Autodesk Inventor part; units mm, degrees
ref_plane "YZ Plane" through (0, 0, 0) normal (1, 0, 0) x (0, 1, 0)
ref_plane "XZ Plane" through (0, 0, 0) normal (0, 1, 0) x (-1, 0, 0)
ref_plane "XY Plane" through (0, 0, 0) normal (0, 0, 1) x (1, 0, 0)
sketch "Sketch1" plane through (0, 0, 0) normal (0, 0, 1) x (1, 0, 0)
  circle A0 centre (0, 0) radius 3.5
  line L0 (77.9423, 0) -> (38.9711, -67.5)
  line L1 (38.9711, -67.5) -> (-38.9711, -67.5)
  line L2 (-38.9711, -67.5) -> (-77.9423, 0)
  line L3 (-77.9423, 0) -> (-38.9711, 67.5)
  line L4 (-38.9711, 67.5) -> (38.9711, 67.5)
  line L5 (38.9711, 67.5) -> (77.9423, 0)
  circle A1 centre (22.5, 0) radius 2.25
  circle A2 centre (54, 0) radius 2
  circle A3 centre (15.9099, 15.9099) radius 2.25
  circle A4 centre (0, 22.5) radius 2.25
  circle A5 centre (-15.9099, 15.9099) radius 2.25
  circle A6 centre (-22.5, 0) radius 2.25
  circle A7 centre (-15.9099, -15.9099) radius 2.25
  circle A8 centre (0, -22.5) radius 2.25
  circle A9 centre (15.9099, -15.9099) radius 2.25
  circle A10 centre (46.7654, 27) radius 2
  circle A11 centre (27, 46.7654) radius 2
  circle A12 centre (0, 54) radius 2
  circle A13 centre (-27, 46.7654) radius 2
  circle A14 centre (-46.7654, 27) radius 2
  circle A15 centre (-54, 0) radius 2
  circle A16 centre (-46.7654, -27) radius 2
  circle A17 centre (-27, -46.7654) radius 2
  circle A18 centre (0, -54) radius 2
  circle A19 centre (27, -46.7654) radius 2
  circle A20 centre (46.7654, -27) radius 2
  dimension "d0" = 7
  dimension "d1" = 135
  dimension "d2" = 22.5
  dimension "d3" = 4.5
  dimension "d4" = 4
  dimension "d5" = 54
  dimension "d8" = 360
  dimension "d12" = 360
extrude "Extrusion1" add sketch "Sketch1" along normal blind 30
sketch "Sketch2" plane through (0, 0, 30) normal (0, 0, 1) x (1, 0, 0)
  circle A0 centre (0, 0) radius 3.5
  circle A1 centre (0, 0) radius 49
  dimension "d16" = 98
extrude "Extrusion2" cut sketch "Sketch2" against normal blind 15
sketch "Sketch3" plane through (0, 0, 15) normal (0, 0, 1) x (1, 0, 0)
  circle A0 centre (0, 0) radius 33
  dimension "d19" = 66
extrude "Extrusion3" cut sketch "Sketch3" against normal blind 3
sketch "Sketch4" plane through (0, 0, 12) normal (0, 0, 1) x (1, 0, 0)
  circle A0 centre (0, 0) radius 16.5
  circle A1 centre (0, 0) radius 3.5
  dimension "d22" = 33
extrude "Extrusion4" add sketch "Sketch4" along normal blind 33
sketch "Sketch5" plane through (0, 0, 45) normal (0, 0, 1) x (1, 0, 0)
  circle A0 centre (8, 0) radius 2.5
  circle A1 centre (2.4721, 7.6085) radius 2.5
  circle A2 centre (-6.4721, 4.7023) radius 2.5
  circle A3 centre (-6.4721, -4.7023) radius 2.5
  circle A4 centre (2.4721, -7.6085) radius 2.5
  point P0 (0, 0)
  dimension "d25" = 5
  dimension "d26" = 8
  dimension "d29" = 360
extrude "Extrusion5" cut sketch "Sketch5" against normal through all
sketch "Sketch6" plane through (0, 0, 0) normal (0, 0, -1) x (-1, 0, 0)
  circle A0 centre (0, 0) radius 17.5
  dimension "d33" = 35
extrude "Extrusion6" cut sketch "Sketch6" against normal blind 5
sketch "Sketch10" plane through (0, 0, 0) normal (0, 0, -1) x (-1, 0, 0)
  circle A0 centre (22.5, 0) radius 2.25
  circle A1 centre (0, 0) radius 3.5
  circle A2 centre (0, 0) radius 20.25
  circle A3 centre (0, 0) radius 24.75
  circle A4 centre (0, 0) radius 16
  circle A5 centre (0, 0) radius 29
  line L0 (29, 0) -> (16, 0)
  dimension "d38" = 13
extrude "Extrusion7" cut sketch "Sketch10" against normal blind 5 contours L0 A0 | A2 | A3 | A5 | A0 L0
sketch "Sketch11" plane through (0, 0, 12) normal (0, 0, 1) x (1, 0, 0)
  circle A0 centre (0, 0) radius 16.5
  circle A1 centre (15.9099, -15.9099) radius 2.25
  circle A2 centre (0, -22.5) radius 2.25
  circle A3 centre (-15.9099, -15.9099) radius 2.25
  circle A4 centre (-22.5, 0) radius 2.25
  circle A5 centre (-15.9099, 15.9099) radius 2.25
  circle A6 centre (0, 22.5) radius 2.25
  circle A7 centre (15.9099, 15.9099) radius 2.25
  circle A8 centre (22.5, 0) radius 2.25
  circle A9 centre (0, 0) radius 33
extrude "Extrusion8" add sketch "Sketch11" along normal up to surface (3 mm away) from surface at 0
sketch "Sketch12" plane through (0, 0, 30) normal (0, 0, 1) x (1, 0, 0)
  circle A0 centre (0, 0) radius 49
  circle A1 centre (46.7654, -27) radius 2
  circle A2 centre (27, -46.7654) radius 2
  circle A3 centre (0, -54) radius 2
  circle A4 centre (-27, -46.7654) radius 2
  circle A5 centre (-46.7654, -27) radius 2
  circle A6 centre (-54, 0) radius 2
  circle A7 centre (-46.7654, 27) radius 2
  circle A8 centre (-27, 46.7654) radius 2
  circle A9 centre (0, 54) radius 2
  circle A10 centre (27, 46.7654) radius 2
  circle A11 centre (46.7654, 27) radius 2
  circle A12 centre (54, 0) radius 2
  line L0 (38.9711, -67.5) -> (77.9423, 0)
  line L1 (77.9423, 0) -> (38.9711, 67.5)
  line L2 (38.9711, 67.5) -> (-38.9711, 67.5)
  line L3 (-38.9711, 67.5) -> (-77.9423, 0)
  line L4 (-77.9423, 0) -> (-38.9711, -67.5)
  line L5 (-38.9711, -67.5) -> (38.9711, -67.5)
extrude "Extrusion9" cut sketch "Sketch12" against normal blind 1
sketch "Sketch14" plane through (0, 0, 15) normal (0, 0, 1) x (1, 0, 0)
  circle A0 centre (0, 0) radius 3.5
  circle A1 centre (0, 0) radius 33
  circle A2 centre (15.9099, -15.9099) radius 2.25
  circle A3 centre (0, -22.5) radius 2.25
  circle A4 centre (-15.9099, -15.9099) radius 2.25
  circle A5 centre (-22.5, 0) radius 2.25
  circle A6 centre (-15.9099, 15.9099) radius 2.25
  circle A7 centre (0, 22.5) radius 2.25
  circle A8 centre (15.9099, 15.9099) radius 2.25
  circle A9 centre (22.5, 0) radius 2.25
  circle A10 centre (0, 0) radius 16.5
  circle A11 centre (0, 0) radius 49
  dimension "d45" = 66
extrude "Extrusion10" cut sketch "Sketch14" against normal blind 4 contours A11
sketch "Sketch15" plane through (0, 0, 29) normal (0, 0, 1) x (1, 0, 0)
  circle A0 centre (0, 0) radius 49 construction
  circle A1 centre (54, 0) radius 2 construction
  circle A2 centre (46.7654, 27) radius 2 construction
  circle A3 centre (27, 46.7654) radius 2 construction
  circle A4 centre (0, 54) radius 2 construction
  circle A5 centre (-27, 46.7654) radius 2 construction
  circle A6 centre (-46.7654, 27) radius 2 construction
  circle A7 centre (-54, 0) radius 2 construction
  circle A8 centre (-46.7654, -27) radius 2 construction
  circle A9 centre (-27, -46.7654) radius 2 construction
  circle A10 centre (0, -54) radius 2 construction
  circle A11 centre (27, -46.7654) radius 2 construction
  circle A12 centre (46.7654, -27) radius 2 construction
  line L0 (77.9423, 0) -> (38.9711, -67.5)
  line L1 (38.9711, 67.5) -> (77.9423, 0)
  line L2 (-38.9711, 67.5) -> (38.9711, 67.5)
  line L3 (-77.9423, 0) -> (-38.9711, 67.5)
  line L4 (-38.9711, -67.5) -> (-77.9423, 0)
  line L5 (38.9711, -67.5) -> (-38.9711, -67.5)
  line L6 (36.0844, 62.5) -> (72.1688, 0)
  line L7 (72.1688, 0) -> (36.0844, -62.5)
  line L8 (36.0844, -62.5) -> (-36.0844, -62.5)
  line L9 (-36.0844, -62.5) -> (-72.1688, 0)
  line L10 (-72.1688, 0) -> (-36.0844, 62.5)
  line L11 (-36.0844, 62.5) -> (36.0844, 62.5)
  dimension "d48" = 5
extrude "Extrusion11" add sketch "Sketch15" along normal blind 0.8
sketch "Sketch16" plane through (0, 0, 0) normal (0, 0, -1) x (-1, 0, 0)
  circle A0 centre (0, 0) radius 29
  circle A1 centre (-46.7654, -27) radius 2
  circle A2 centre (-27, -46.7654) radius 2
  circle A3 centre (0, -54) radius 2
  circle A4 centre (27, -46.7654) radius 2
  circle A5 centre (46.7654, -27) radius 2
  circle A6 centre (54, 0) radius 2
  circle A7 centre (46.7654, 27) radius 2
  circle A8 centre (27, 46.7654) radius 2
  circle A9 centre (0, 54) radius 2
  circle A10 centre (-27, 46.7654) radius 2
  circle A11 centre (-46.7654, 27) radius 2
  circle A12 centre (-54, 0) radius 2
  line L0 (-77.9423, 0) -> (-38.9711, -67.5)
  line L1 (-38.9711, -67.5) -> (38.9711, -67.5)
  line L2 (38.9711, -67.5) -> (77.9423, 0)
  line L3 (77.9423, 0) -> (38.9711, 67.5)
  line L4 (38.9711, 67.5) -> (-38.9711, 67.5)
  line L5 (-38.9711, 67.5) -> (-77.9423, 0)
  line L6 (68.1273, 0) -> (34.0637, -59)
  line L7 (34.0637, -59) -> (-34.0637, -59)
  line L8 (-34.0637, -59) -> (-68.1273, 0)
  line L9 (-68.1273, 0) -> (-34.0637, 59)
  line L10 (-34.0637, 59) -> (34.0637, 59)
  line L11 (34.0637, 59) -> (68.1273, 0)
  dimension "d51" = 118
extrude "Extrusion12" cut sketch "Sketch16" along normal through all both and the other way through all contours L5 L4 L3 L2 L1 L0
sketch "Sketch17" plane through (0, 0, 0) normal (0, 0, -1) x (-1, 0, 0)
  circle A0 centre (0, -54) radius 2
  circle A1 centre (0, -54) radius 2
  circle A2 centre (27, -46.7654) radius 2
  circle A3 centre (46.7654, -27) radius 2
  circle A4 centre (54, 0) radius 2
  circle A5 centre (46.7654, 27) radius 2
  circle A6 centre (27, 46.7654) radius 2
  circle A7 centre (0, 54) radius 2
  circle A8 centre (-27, 46.7654) radius 2
  circle A9 centre (-46.7654, 27) radius 2
  circle A10 centre (-54, 0) radius 2
  circle A11 centre (-46.7654, -27) radius 2
  circle A12 centre (-27, -46.7654) radius 2
  point P0 (0, 0)
  dimension "d56" = 360
extrude "Extrusion13" add sketch "Sketch17" along normal up to surface (29 mm away) from surface at -29
sketch "Sketch18" plane through (0, 0, 0) normal (0, 0, -1) x (-1, 0, 0)
  line L0 (-46.188, 0) -> (-23.094, 40)
  line L1 (-23.094, 40) -> (23.094, 40)
  line L2 (23.094, 40) -> (46.188, 0)
  line L3 (46.188, 0) -> (23.094, -40)
  line L4 (23.094, -40) -> (-23.094, -40)
  line L5 (-23.094, -40) -> (-46.188, 0)
  line L6 (-19.0526, -33) -> (19.0526, -33)
  line L7 (19.0526, -33) -> (38.1051, 0)
  line L8 (38.1051, 0) -> (19.0526, 33)
  line L9 (19.0526, 33) -> (-19.0526, 33)
  line L10 (-19.0526, 33) -> (-38.1051, 0)
  line L11 (-38.1051, 0) -> (-19.0526, -33)
  line L12 (-34.0637, -59) -> (34.0637, -59)
  line L13 (34.0637, -59) -> (68.1273, 0)
  line L14 (68.1273, 0) -> (34.0637, 59)
  line L15 (34.0637, 59) -> (-34.0637, 59)
  line L16 (-34.0637, 59) -> (-68.1273, 0)
  line L17 (-68.1273, 0) -> (-34.0637, -59)
  circle A0 centre (0, 0) radius 29
  dimension "d60" = 80
  dimension "d61" = 7
extrude "Extrusion14" add sketch "Sketch18" along normal blind 13 contours L0 L1 L2 L3 L4 L5 | L17 L16 L15 L14 L13 L12
sketch "Sketch19" plane through (68.1273, 0, 29) normal (0.866, 0.5, 0) x (0, 0, -1)
  line L0 (29, 15.0111) -> (29, 53.1162)
  line L1 (29, 15.0111) -> (42, 15.0111)
  line L2 (42, 53.1162) -> (42, 15.0111)
  line L3 (29, 53.1162) -> (42, 53.1162)
  line L4 (38, 26.9926) -> (33, 41.1347) construction
  circle A0 centre (38, 26.9926) radius 2.5
  circle A1 centre (33, 41.1347) radius 2.5
  point P0 (29, 34.0637)
  point P1 (35.5, 15.0111)
  point P2 (35.5, 34.0637)
  point P3 (29, 34.0637)
  dimension "d64" = 15
  dimension "d65" = 5
  dimension "d66" = 5
  dimension "d72" = 5
extrude "Extrusion15" cut sketch "Sketch19" against normal blind 30 contours A0 | A1
pattern_circular "Circular Pattern1" count 6 over 360 about axis through (0, 0, 0) along (0, 0, 1) of "Extrusion15"
sketch "Sketch21" plane through (0, 0, 5) normal (0, 0, -1) x (-1, 0, 0)
  circle A0 centre (0, 17.5) radius 2
  circle A1 centre (-15.1554, -8.75) radius 2
  circle A2 centre (15.1554, -8.75) radius 2
  point P0 (0, 0)
  dimension "d74" = 4
  dimension "d75" = 17.5
  dimension "d78" = 360
extrude "Extrusion16" cut sketch "Sketch21" against normal through all
sketch "Sketch22" plane through (0, 0, 5) normal (0, 0, -1) x (-1, 0, 0)
  circle A0 centre (-15.1554, -8.75) radius 2
  circle A1 centre (0, 17.5) radius 2
  circle A2 centre (15.1554, -8.75) radius 2
  circle A3 centre (0, 0) radius 29
  circle A4 centre (-22.5, 0) radius 2.25
  circle A5 centre (-15.9099, 15.9099) radius 2.25
  circle A6 centre (0, 22.5) radius 2.25
  circle A7 centre (15.9099, 15.9099) radius 2.25
  circle A8 centre (22.5, 0) radius 2.25
  circle A9 centre (15.9099, -15.9099) radius 2.25
  circle A10 centre (0, -22.5) radius 2.25
  circle A11 centre (-15.9099, -15.9099) radius 2.25
  circle A12 centre (0, 0) radius 3.5
extrude "Extrusion17" cut sketch "Sketch22" against normal blind 5
sketch "Sketch23" plane through (0, 0, 10) normal (0, 0, -1) x (-1, 0, 0)
  circle A0 centre (0, 0) radius 3.5
  circle A1 centre (0, 0) radius 13.5
  dimension "d84" = 27
extrude "Extrusion18" cut sketch "Sketch23" against normal blind 7
sketch "Sketch24" plane through (0, 0, 29) normal (0, 0, 1) x (1, 0, 0)
  line L0 (-34.0637, -59) -> (34.0637, -59)
  line L1 (34.0637, -59) -> (68.1273, 0)
  line L2 (68.1273, 0) -> (34.0637, 59)
  line L3 (34.0637, 59) -> (-34.0637, 59)
  line L4 (-34.0637, 59) -> (-68.1273, 0)
  line L5 (-68.1273, 0) -> (-34.0637, -59)
  circle A0 centre (0, 0) radius 49
extrude "Extrusion19" add sketch "Sketch24" along normal blind 1
properties part number "AC05" material "ABS Plastic"
Check sheet for the modelled part. Datum: model origin and axes. Units: mm. A direction names the side the tool comes from. Coordinates: 2 decimals unless noted, no trailing zeros. Loops run counter-clockwise (first coordinate to the right, second up) from the corner with the lowest first, then second, coordinate; pieces in that order, holes last. Notation, with made-up numbers: (42.25, -33) -> (68.25, -33) arc R19 ccw to (68.25, -13) -> close; hole circle Ø11 at (12.5, 48.25). An arc over 180 degrees is marked (long way). Write item = value, one per line. Start each with the question number.
1. Depth check by flat-ended pin: P1, Ø2, axis at x = -51, y = 35, coming from the +Z side; P2, Ø2, axis at y = 34, z = 4.5, coming from the -X side; P3, Ø1.5, axis at x = 8.5, y = -25, coming from the -Z side; P4, Ø2, axis at x = 38.5, y = -28, coming from the +Z side. Enter the tip coordinate at first touch or a pass-through.
2. Section check A-A on z = 23. Give the number of separate pieces and of enclosed holes in the cut face, then the cut area to 3 significant figures.
3. Draft check along Y on faces 1 (the cylindrical face through (-14.7, 14.013, 12.465)), 2 (the flat face through (50.86, -29.91, 8.2)), 3 (the cylindrical face through (-7.822, 46.182, -6.385)). Enter one of: released by +Y, released by -Y, zero draft, split by the parting line, or undercut.
4. Tool access check on faces 4 (the flat face through (-8, 15, 15)), 5 (the cylindrical face through (9.51, 46.18, -8.46)), 6 (the flat face through (-28.71, 16.27, -6.41)), 7 (the cylindrical face through (15.62, 13.68, 12.46)). Record the directions out of +Z, -Z, +X, -X, +Y, -Y that give a thin tool (end or side, any length) a straight path to the whole face; none if there is none.
5. Material ranges on line 1 (Y direction, x = 0, z = 3); line 2 (Y direction, x = -43, z = -3); line 3 (Y direction, x = -7, z = 28), recorded low to high.
6. Section check B-B on z = 8. Record the cut outline in (x, y).
Responses:
q1.P1 = through
q1.P2 = -49.07
q1.P3 = 10
q1.P4 = 11
q2.separate_pieces = 2
q2.enclosed_holes = 7
q2.area = 5,230 mm2
q3.face_1 = undercut
q3.face_2 = released by -Y
q3.face_3 = zero draft
q4.face_4 = +Z
q4.face_5 = +Y
q4.face_6 = -Z
q4.face_7 = +Z, -Z
q5.line_1 = -59 to -29, 29 to 59
q5.line_2 = -43.52 to -35.64, -30.35 to 14.02, 19.31 to 43.52
q5.line_3 = -59 to -48.5, -14.94 to -7.15, -2.26 to 2.26, 7.15 to 14.94, 48.5 to 59
q6.outline = (-68.13, 0) -> (-34.06, -59) -> (34.06, -59) -> (68.13, 0) -> (34.06, 59) -> (-34.06, 59) -> close; hole circle Ø58 at (0, 0)
